Could you check a few things on this drawing? It's one solid part, dimensions in mm from its lowest x, y, z. Give positions to 0.01 mm unless a question says otherwise; leave off trailing zeros. Loops run counter-clockwise (first coordinate to the right, second up) from the corner with the lowest first, then second, coordinate; pieces in that order, holes last. Notation, with made-up numbers: M -23,67 L 28,67 A25 cw 28,83 Z; hole C -3.5,74.25 d2. An arc over 180 degrees is marked long. Return JSON: item names as keys, results as strings. Group by question number.
1. If we section it at A-A (y = 44): Write out the boundary of the cut face in (x, z) (1 decimal).
2. If we section it at C-C (z = 8): Write out the boundary of the cut face in (x, y) (1 decimal).
3. Please list where these lines run through material, in increasing order: line 1 (X direction, y = 37, z = 25) (1 decimal); line 2 (Z direction, x = 29.5, y = 17) (1 decimal); line 3 (Z direction, x = 29, y = 37.5).
4. For pin 1 (8 mm diameter, centred on y = 34.5, z = 12, fed in from +X) (1 decimal); pin 2 (5 mm diameter, centred on y = 21.5, z = 15, fed in from +X); pin 3 (12 mm diameter, centred on x = 12.5, y = 33.5, fed in from +Z) (1 decimal), each with a flat end and sliding along its axis, tell me the tip position at first contact or that it passes through.
5. If we section it at B-B (x = 4): Write out the boundary of the cut face in (y, z) (1 decimal).
6. If we mould it in two halves opening along Z, with no side actions, what happens to the marked faces 1, 2 and 3? For each: +Z half, -Z half, draft (parallel to the pull), parting line (faces both ways), or undercut.
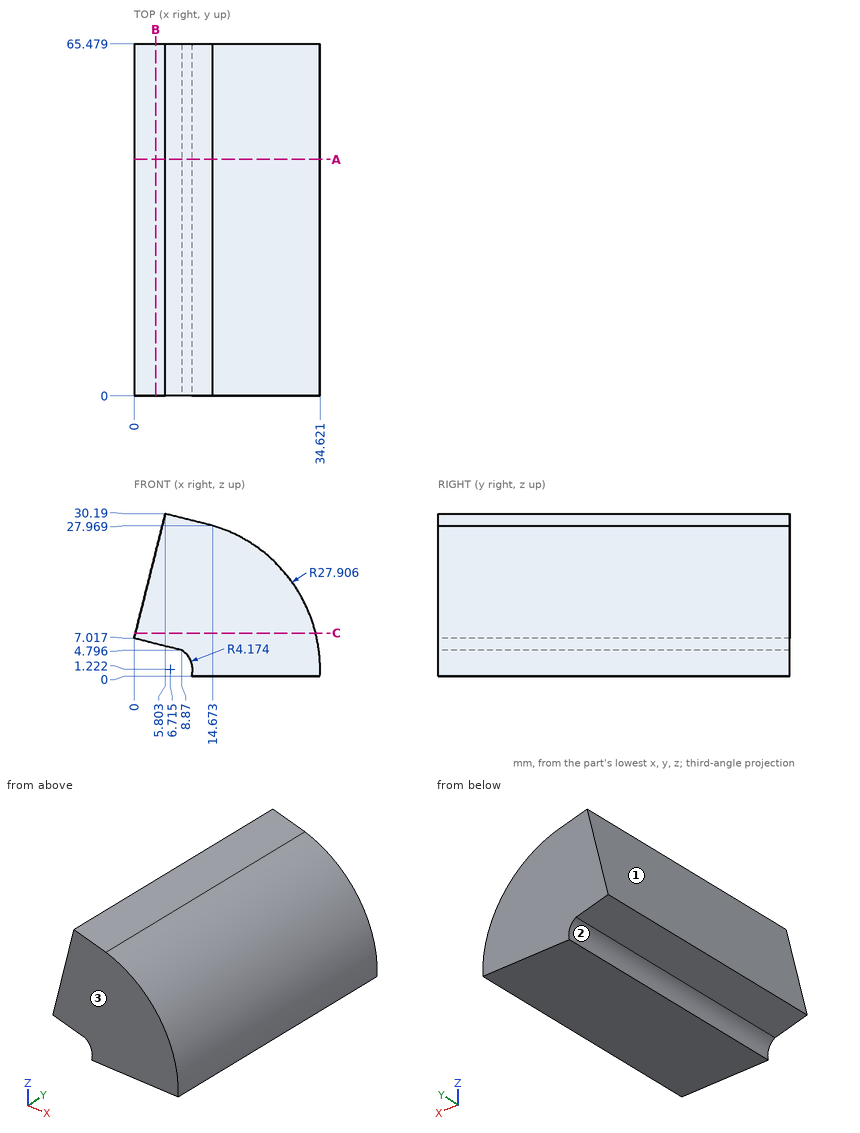
Answer:
{
 "1": {"outline": "M 0,7 L 8.9,4.8 A4.2 cw 10.7,0 L 34.6,0 A27.9 ccw 14.7,28 L 5.8,30.2 Z"},
 "2": {"outline": "M 0.2,0 L 33.8,0 L 33.8,65.5 L 0.2,65.5 Z"},
 "3": {"line 1": "x = 4.5 to 21.3", "line 2": "z = 0 to 17.3", "line 3": "z = 0 to 18.02"},
 "4": {"pin 1": "stops at x = 33.8", "pin 2": "stops at x = 32.24", "pin 3": "stops at z = 30"},
 "5": {"outline": "M 0,6 L 65.5,6 L 65.5,23 L 0,23 Z"},
 "6": {"face 1": "+Z half", "face 2": "undercut", "face 3": "draft"}
}
